```python
from build123d import *

# Parameters (mm, degrees)
F1_DEPTH = 7
F2_W     = 15
F2_H     = 7
F2_R     = 1.75
F3_DEPTH = 7
F4_R     = 2.5
F5_DEPTH = 10


with BuildPart() as f1:
    # F0 (on Top) → F1 (new body)
    with BuildSketch(Plane.XY):
        with BuildLine():
            ThreePointArc((27.5, 22.5), (26.035534, 26.035534), (22.5, 27.5))
            Line((22.5, 27.5), (-22.5, 27.5))
            ThreePointArc((-22.5, 27.5), (-26.035534, 26.035534), (-27.5, 22.5))
            Line((-27.5, 22.5), (-27.5, -22.5))
            ThreePointArc((-27.5, -22.5), (-26.035534, -26.035534), (-22.5, -27.5))
            Line((-22.5, -27.5), (22.5, -27.5))
            ThreePointArc((22.5, -27.5), (26.035534, -26.035534), (27.5, -22.5))
            Line((27.5, -22.5), (27.5, 22.5))
        make_face()
    extrude(amount=F1_DEPTH)

    # F2 (on face) → F3 (join)
    with BuildSketch(Plane.XY.offset(7)):
        Rectangle(F2_W, F2_H)
        with Locations((-4.5, 0)):
            Circle(F2_R, mode=Mode.SUBTRACT)
        with BuildLine():
            ThreePointArc((6.25, 0), (4.5, -1.75), (2.75, 0))
            ThreePointArc((2.75, 0), (4.5, 1.75), (6.25, 0))
        make_face(mode=Mode.SUBTRACT)
    extrude(amount=F3_DEPTH)

    # F4 (on face) → F5 (cut)
    with BuildSketch(Plane(origin=(0, 0, 0), x_dir=(1, 0, 0), z_dir=(0, 0, -1))):
        with Locations((-4.5, 0)):
            Circle(F4_R)
        with BuildLine():
            ThreePointArc((7, 0), (4.5, 2.5), (2, 0))
            ThreePointArc((2, 0), (4.5, -2.5), (7, 0))
        make_face()
    extrude(amount=-F5_DEPTH, mode=Mode.SUBTRACT)


solid = f1.part
```
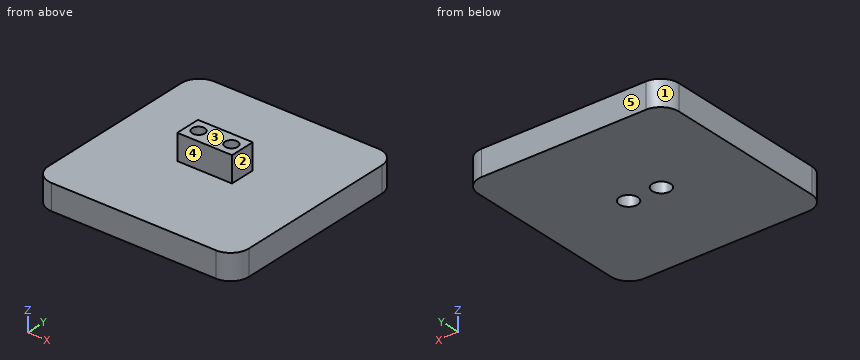
Here's how the part is built. I have some questions about the finished solid (model axes, mm). Face numbers are marked on the shaded views. A direction names the side the tool comes from. Coordinates: 2 decimals unless noted, no trailing zeros. Write each loop counter-clockwise with the first axis right and the second up, starting at its lowest first coordinate (ties: lowest second). Pieces come first, ordered by that corner, then holes. Notation, with made-up numbers: M -14,15 L 7,15 A4 cw 7,22 Z; hole C 68,4 d2. An arc over 180 degrees is marked long. Answer as CSV lines item,"result". Start each with the question number.
Q1. Suppose I cut it at B-B, the plane z = 2.5. List the corners of the cut face in (x, y) for me.
Q2. Will these pins go through, and if not, where does the flat tip stop? pin 1 Ø3 at (y, z) = (-19.5, 7.5) entering from -X; pin 2 Ø1.5 at (x, y) = (7, -19) entering from +Z; pin 3 Ø5.5 at (y, z) = (-1, 10.5) entering from +X; pin 4 Ø7.5 at (x, z) = (0, 11) entering from -Y.
Q3. Suppose I cut it at D-D, the plane z = 11. List the corners of the cut face in (x, y) for me.
Q4. If we mould it in two halves opening along Y, with no side actions, what happens to the marked faces 3, 4 and 5? For each: pulls with the +Y half, pulls with the -Y half, needs draft (parallel to the pull), parting line crosses it, or undercut.
Q5. Suppose I cut it at A-A, the plane x = 4.5. List the corners of the cut face in (y, z) for me, then the cut area to 3 significant figures.
Q6. I need wall thicknesses on probe 1 along Y at (x, z) = (-4.5, 13.05); probe 2 along Y at (x, z) = (-4.5, 3.5); probe 3 along X at (y, z) = (1.5, 3.25). Which ranges of each line are inside material? Lowest first, please. Write a range as [from, to].
Q7. Suppose I cut it at C-C, the plane y = 0. List the corners of the cut face in (x, z) for me, then the cut area to 3 significant figures.
Q8. For the marked faces 1 and 2, which set-ups out of +Z, -Z, +X, -X, +Y, -Y let a thin tool reach every point of the face, with its end or its side?
Entries:
1,outline,"M -27.5,-22.5 A5 ccw -22.5,-27.5 L 22.5,-27.5 A5 ccw 27.5,-22.5 L 27.5,22.5 A5 ccw 22.5,27.5 L -22.5,27.5 A5 ccw -27.5,22.5 Z; hole C -4.5,0 d5; hole C 4.5,0 d5"
2,pin 1,"stops at x = -27.5"
2,pin 2,"stops at z = 7"
2,pin 3,"stops at x = 7.5"
2,pin 4,"stops at y = -3.5"
3,outline,"M -7.5,-3.5 L 7.5,-3.5 L 7.5,3.5 L -7.5,3.5 Z; hole C -4.5,0 d3.5; hole C 4.5,0 d3.5"
4,face 3,"needs draft"
4,face 4,"pulls with the -Y half"
4,face 5,"pulls with the +Y half"
5,outline,"M -27.5,0 L -2.5,0 L -2.5,10 L -1.75,10 L -1.75,14 L -3.5,14 L -3.5,7 L -27.5,7 Z; M 1.75,10 L 2.5,10 L 2.5,0 L 27.5,0 L 27.5,7 L 3.5,7 L 3.5,14 L 1.75,14 Z"
5,area,"370 mm²"
6,probe 1,"y = [-3.5, -1.75], [1.75, 3.5]"
6,probe 2,"y = [-27.5, -2.5], [2.5, 27.5]"
6,probe 3,"x = [-27.5, -6.5], [-2.5, 2.5], [6.5, 27.5]"
7,outline,"M -27.5,0 L -7,0 L -7,10 L -6.25,10 L -6.25,14 L -7.5,14 L -7.5,7 L -27.5,7 Z; M -2.75,10 L -2,10 L -2,0 L 2,0 L 2,10 L 2.75,10 L 2.75,14 L -2.75,14 Z; M 6.25,10 L 7,10 L 7,0 L 27.5,0 L 27.5,7 L 7.5,7 L 7.5,14 L 6.25,14 Z"
7,area,"362 mm²"
8,face 1,"+Z, -Z, -X, +Y"
8,face 2,"+Z, +X, +Y, -Y"
